Part print with two shaded views. Sizes in mm from the minimum x, y, z corner. Give positions to 0.01 mm unless a question says otherwise; leave off trailing zeros. Write each loop counter-clockwise with the first axis right and the second up, starting at its lowest first coordinate (ties: lowest second). Pieces come first, ordered by that corner, then holes.
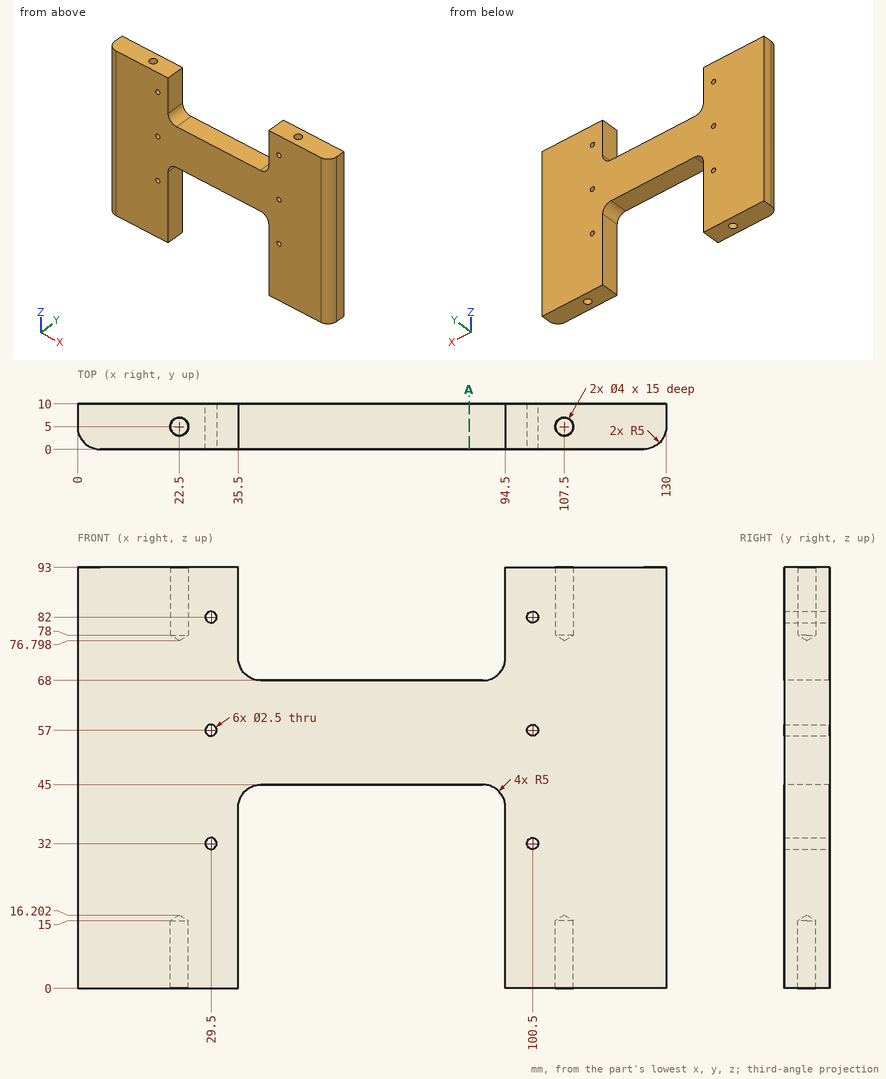
1) Drill centre lines: L1, parallel to X at y = 5, z = 86.5; L2, parallel to Z at x = 29.5, y = 6.75; L3, parallel to Y at x = 22.5, z = 9.75. Where is each one in solid material? Low to high.
Check result:
L1: x = 0 to 20.5, 24.5 to 35.5, 94.5 to 105.5, 109.5 to 130
L2: z = 0 to 30.75, 33.25 to 55.75, 58.25 to 80.75, 83.25 to 93
L3: y = 0 to 3, 7 to 10
2) Flat gauge pins, fed straight in: P1, Ø2, axis at x = 44.5, y = 5, coming from the -Z side; P2, Ø3, axis at x = 100.5, z = 57, coming from the +Y side; P3, Ø3, axis at x = 107.5, y = 5, coming from the -Z side; P4, Ø3.5, axis at x = 107.5, y = 5, coming from the -Z side. Where does each tip first touch, or does it go through?
Check result:
P1: stops at z = 45
P2: stops at y = 10
P3: stops at z = 15.3
P4: stops at z = 15.15
3) Saw through at A-A (x = 86.5). Write the cut outline in (y, z).
Check result:
outline: (0, 45) - (10, 45) - (10, 68) - (0, 68) - close
